```python
from build123d import *

# Parameters (mm, degrees)
SKETCH1_R           = 3
BOSS_EXTRUDE1_DEPTH = 0.4
SKETCH2_R           = 2.5
BOSS_EXTRUDE2_DEPTH = 8.6
SHELL1_START        = -8.5
SHELL1_OUTLINE_R    = 2
SHELL1_DEPTH        = 8.5
CUT_EXTRUDE1_REACH  = 11.95
SKETCH3_R           = 1.5


# Read off the part's stored shape, not the designer's step: Shell1
with BuildPart() as part:
    # Sketch1 → Boss-Extrude1 (new body)
    with BuildSketch(Plane(origin=(0, 0, 0), x_dir=(1, 0, 0), z_dir=(0, 1, 0))):
        with Locations(Location((0, 0, 0), (0, 0, 270))):
            Circle(SKETCH1_R)
    extrude(amount=-BOSS_EXTRUDE1_DEPTH)

    # Sketch2 → Boss-Extrude2 (add)
    with BuildSketch(Plane.XZ.offset(0.4)):
        with Locations(Location((0, 0, 0), (0, 0, 90))):
            Circle(SKETCH2_R)
    extrude(amount=BOSS_EXTRUDE2_DEPTH)

    # Shell1 outline → Shell1 (cut)
    with BuildSketch(Plane(origin=(0, 0, 0), x_dir=(1, 0, 0), z_dir=(0, 1, 0)).offset(SHELL1_START)):
        Circle(SHELL1_OUTLINE_R)
    extrude(amount=SHELL1_DEPTH, mode=Mode.SUBTRACT)

    # Sketch3 → Cut-Extrude1 (cut, up to next)
    with BuildSketch(Plane.XZ.offset(9), mode=Mode.PRIVATE) as cut_extrude1_sk1:
        with Locations(Location((0, 0, 0), (0, 0, 270))):
            Circle(SKETCH3_R)
    cut_extrude1_tool1 = extrude(cut_extrude1_sk1.sketch, amount=-CUT_EXTRUDE1_REACH, mode=Mode.PRIVATE) & part.part
    add(cut_extrude1_tool1.solids().sort_by_distance((0, -9, 0))[0], mode=Mode.SUBTRACT)


solid = part.part
```
Could you check a few things on this model? Use its own coordinates, in mm. A direction names the side the tool comes from. Round coordinates to 2 decimals unless told otherwise and drop trailing zeros. Order: outer loops, then holes, each group sorted by start corner. A loop starts at its lowest first (then second) coordinate and runs counter-clockwise, first axis right, second up. Notation, with made-up numbers: (8.25, 46) -> (39.25, 46) arc R14 ccw to (39.25, 73) -> close; hole circle Ø9 at (35.25, 58). An arc over 180 degrees is marked (long way). One line per question, with ' | ' between items.
Q1. I'm going to push a flat-ended pin straight in: pin 1 (2 mm diameter, centred on x = -1, y = -7, fed in from +Z). Where does the tip first touch, or does it pass through?
Computed values:
pin 1: z = 2.5
Q2. Which directions (+Z, -Z, +X, -X, +Y, -Y) give clear straight access to the entire face, cutting with the end or side of a thin tool? Please do faces 4 (the face through (0, -4, 2)), 5 (the face through (0.9, -0.2, 2.86)).
Computed values:
face 4: +Y | face 5: +Y, -Y
Q3. If we section it at A-A on z = 0: Write out the boundary of the cut face in (x, y), plus the area to 3 significant figures.
Computed values:
outline: (-3, -0.4) -> (-2.5, -0.4) -> (-2.5, -9) -> (-1.5, -9) -> (-1.5, -8.5) -> (-2, -8.5) -> (-2, 0) -> (-3, 0) -> close; (1.5, -9) -> (2.5, -9) -> (2.5, -0.4) -> (3, -0.4) -> (3, 0) -> (2, 0) -> (2, -8.5) -> (1.5, -8.5) -> close | area: 9.90 mm²
Q4. If we section it at B-B on x = 0: Write out the boundary of the cut face in (y, z), plus the area to 3 significant figures.
Computed values:
outline: (-9, -2.5) -> (-0.4, -2.5) -> (-0.4, -3) -> (0, -3) -> (0, -2) -> (-8.5, -2) -> (-8.5, -1.5) -> (-9, -1.5) -> close; (-9, 1.5) -> (-8.5, 1.5) -> (-8.5, 2) -> (0, 2) -> (0, 3) -> (-0.4, 3) -> (-0.4, 2.5) -> (-9, 2.5) -> close | area: 9.90 mm²
Q5. If we section it at C-C on y = -6.5: Write out the boundary of the cut face in (x, z), plus the area to 3 significant figures.
Computed values:
outline: circle Ø5 at (0, 0); hole circle Ø4 at (0, 0) | area: 7.07 mm²
Q6. If we section it at D-D on x = 2.4: Write out the boundary of the cut face in (y, z), plus the area to 3 significant figures.
Computed values:
outline: (-9, -0.7) -> (-0.4, -0.7) -> (-0.4, -1.8) -> (0, -1.8) -> (0, 1.8) -> (-0.4, 1.8) -> (-0.4, 0.7) -> (-9, 0.7) -> close | area: 13.5 mm²
Q7. We'd pull the mould along X, two halves only. Please class faces 1 (the face through (2, -0.4, -2)), 2 (the face through (2.44, -4.64, -0.54)), 3 (the face through (0.45, -8.75, -1.43)): released by +X, released by -X, zero draft, split by the parting line, or undercut.
Computed values:
face 1: zero draft | face 2: split by the parting line | face 3: undercut
Q8. If I drill on line 1 (X direction, y = -6.25, z = 0); line 2 (X direction, y = -8.75, z = 0); line 3 (Y direction, x = 1.7, z = 2.1), over which ranges is the centre line in solid material (lowest first)? Write a range as from..to.
Computed values:
line 1: -2.5..-2, 2..2.5 | line 2: -2.5..-1.5, 1.5..2.5 | line 3: -0.4..0
